from build123d import *

# Parameters (mm, degrees)
PAD005_DEPTH    = 25
SKETCH012_R     = 2.2
POCKET005_DEPTH = 72.001
SKETCH013_R     = 4.4
POCKET006_DEPTH = 68.001
FILLET003_R     = 1


with BuildPart() as part:
    # Sketch011 → Pad005 (new body, symmetric)
    with BuildSketch(Plane.XY):
        with BuildLine():
            Line((7, 18.3), (34.2, 18.3))
            ThreePointArc((34.2, 18.3), (36, 17.7), (37.8, 18.3))
            Line((37.8, 18.3), (67, 18.3))
            Line((67, 18.3), (67, 16.3))
            Line((67, 16.3), (72, 18.3))
            Line((72, 20.7), (72, 18.3))
            Line((0, 20.7), (72, 20.7))
            Line((0, -20.7), (0, 20.7))
            Line((72, -20.7), (0, -20.7))
            Line((72, -15.7), (72, -20.7))
            Line((67, -13.7), (72, -15.7))
            Line((67, -15.7), (67, -13.7))
            Line((67, -15.7), (7, -15.7))
            Line((7, -15.7), (7, 18.3))
        make_face()
    extrude(amount=PAD005_DEPTH, both=True)

    # Sketch012 → Pocket005 (cut, through all)
    with BuildSketch(Plane.YZ):
        Circle(SKETCH012_R)
    extrude(amount=POCKET005_DEPTH, mode=Mode.SUBTRACT)

    # Sketch013 → Pocket006 (cut, through all)
    with BuildSketch(Plane.YZ.offset(4)):
        Circle(SKETCH013_R)
    extrude(amount=POCKET006_DEPTH, mode=Mode.SUBTRACT)

    # Fillet003
    fillet003_edges = [part.edges().sort_by_distance(p)[0] for p in [
        (36, 20.7, -25),
        (72, 20.7, 0),
        (36, 20.7, 25),
        (36, -20.7, 25),
        (72, -20.7, 0),
        (36, -20.7, -25),
        (72, -15.7, 0),
        (72, 18.3, 0),
        (72, 19.5, -25),
        (72, -18.2, -25),
        (69.5, -14.7, -25),
        (72, -18.2, 25),
        (69.5, 17.3, -25),
        (69.5, 17.3, 25),
        (72, 19.5, 25),
        (69.5, -14.7, 25),
    ]]
    fillet(fillet003_edges, radius=FILLET003_R)


solid = part.part
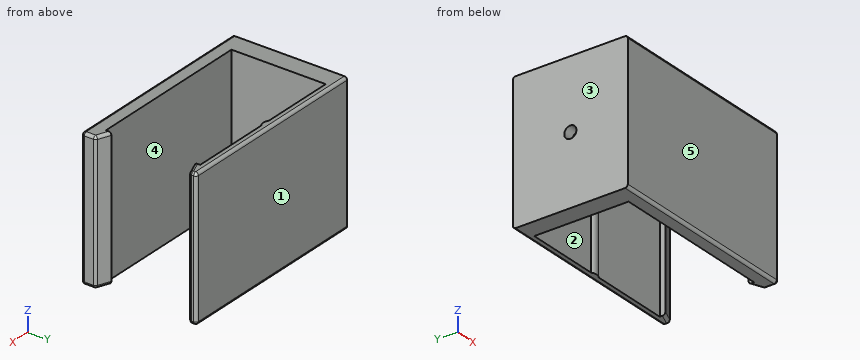
Work out the finished part from the listing and answer in its coordinate system (mm). Face numbers are marked on the shaded views. A direction names the side the tool comes from. Round coordinates to 2 decimals unless told otherwise and drop trailing zeros. Loops run counter-clockwise (first coordinate to the right, second up) from the corner with the lowest first, then second, coordinate; pieces in that order, holes last. Notation, with made-up numbers: (18, 68.5) -> (77, 68.5) arc R14 ccw to (77, 86.5) -> close; hole circle Ø9 at (24, 55). An arc over 180 degrees is marked (long way). Use one line per item in the form item = value.
(1) A tool of negligible diameter and unlimited length cuts with its end or side. For the marked faces 4 and 5, from which of +Z, -Z, +X, -X, +Y, -Y can it reach the whole face along a straight path? Write none if from no direction.
Answer list:
face_4 = +Z, -Z
face_5 = +Z, -Z, +X, -X, -Y
(2) Find section C-C on z = 0. Give the vertices of the cut face in (x, y).
Answer list:
outline = (0, -20.7) -> (71, -20.7) arc R1 ccw to (72, -19.7) -> (72, -16.38) arc R1 ccw to (71.37, -15.45) -> (67, -13.7) -> (67, -15.7) -> (7, -15.7) -> (7, -4.4) -> (4, -4.4) -> (4, -2.2) -> (0, -2.2) -> close; (0, 2.2) -> (4, 2.2) -> (4, 4.4) -> (7, 4.4) -> (7, 18.3) -> (34.2, 18.3) arc R3 ccw to (37.8, 18.3) -> (67, 18.3) -> (67, 16.3) -> (71.37, 18.05) arc R1 ccw to (72, 18.98) -> (72, 19.7) arc R1 ccw to (71, 20.7) -> (0, 20.7) -> close
(3) Find section A-A on x = 17.5. Give the vertices of the cut face in (y, z).
Answer list:
outline = (-20.7, -24) arc R1 ccw to (-19.7, -25) -> (-15.7, -25) -> (-15.7, 25) -> (-19.7, 25) arc R1 ccw to (-20.7, 24) -> close; (18.3, -25) -> (19.7, -25) arc R1 ccw to (20.7, -24) -> (20.7, 24) arc R1 ccw to (19.7, 25) -> (18.3, 25) -> close
(4) Find section B-B on y = 0. Give the vertices of the cut face in (x, z).
Answer list:
outline = (0, -25) -> (7, -25) -> (7, -4.4) -> (4, -4.4) -> (4, -2.2) -> (0, -2.2) -> close; (0, 2.2) -> (4, 2.2) -> (4, 4.4) -> (7, 4.4) -> (7, 25) -> (0, 25) -> close
(5) Find section D-D on z = 22.5. Give the vertices of the cut face in (x, y).
Answer list:
outline = (0, -20.7) -> (71, -20.7) arc R1 ccw to (72, -19.7) -> (72, -16.38) arc R1 ccw to (71.37, -15.45) -> (67, -13.7) -> (67, -15.7) -> (7, -15.7) -> (7, 18.3) -> (34.2, 18.3) arc R3 ccw to (37.8, 18.3) -> (67, 18.3) -> (67, 16.3) -> (71.37, 18.05) arc R1 ccw to (72, 18.98) -> (72, 19.7) arc R1 ccw to (71, 20.7) -> (0, 20.7) -> close
(6) Straight lines are drawn through the part: line 1 (Y direction, x = 11.5, z = 14); line 2 (Y direction, x = 1, z = 0); line 3 (Z direction, x = 1.95, y = 0). For each, find the intervals that lie inside material, in ascending order.
Answer list:
line_1 = -20.7 to -15.7, 18.3 to 20.7
line_2 = -20.7 to -2.2, 2.2 to 20.7
line_3 = -25 to -2.2, 2.2 to 25
(7) Flat-ended cylindrical pins translate along their axes: P1, Ø10, axis at y = -2.5, z = 11, coming from the +X side; P2, Ø2.5, axis at y = 1, z = 0, coming from the +X side. Find the tip coordinate at first contact, or state that the pin passes through.
Answer list:
P1 = 7
P2 = 4
(8) For a pull along Y with two mould halves and no side action, classify the marked faces 1, 2 and 3 as released by +Y, released by -Y, zero draft, split by the parting line, or undercut.
Answer list:
face_1 = released by +Y
face_2 = undercut
face_3 = zero draft
